The model under review builds one solid part; all positions refer to its coordinate system, in mm. A direction names the side the tool comes from. Coordinates: 2 decimals unless noted, no trailing zeros. Order: outer loops, then holes, each group sorted by start corner. A loop starts at its lowest first (then second) coordinate and runs counter-clockwise, first axis right, second up. Notation, with made-up numbers: M -25,23.5 L 4,23.5 A21 ccw 4,31.5 Z; hole C 50,26.5 d4. An arc over 180 degrees is marked long. Answer in a Markdown table with one row per item.
from build123d import *

# Parameters (mm, degrees)
SKETCH_1_W      = 27
SKETCH_1_H      = 27.6
SKETCH_1_W_2    = 23
SKETCH_1_H_2    = 1.5
EXTRUDE_1_DEPTH = 1.6
SKETCH_2_W      = 26.5
SKETCH_2_H      = 15
EXTRUDE_2_DEPTH = 1.5
SKETCH_3_W      = 5.6
SKETCH_3_H      = 12.6
EXTRUDE_3_DEPTH = 2
SKETCH_4_W      = 10.2
SKETCH_4_H      = 2.5
EXTRUDE_4_DEPTH = 2.5


with BuildPart() as part:
    # 草图1 → 凸台-拉伸1 (new body)
    with BuildSketch(Plane(origin=(0, 0, 0), x_dir=(1, 0, 0), z_dir=(0, 1, 0))):
        with Locations((13.5, -13.8)):
            Rectangle(SKETCH_1_W, SKETCH_1_H)
        with Locations((13.5, -26.05)):
            Rectangle(SKETCH_1_W_2, SKETCH_1_H_2, mode=Mode.SUBTRACT)
    extrude(amount=EXTRUDE_1_DEPTH)

    # 草图2 → 凸台-拉伸2 (add)
    with BuildSketch(Plane(origin=(0, 1.6, 0), x_dir=(1, 0, 0), z_dir=(0, 1, 0))):
        with Locations((13.5, -10.5)):
            Rectangle(SKETCH_2_W, SKETCH_2_H)
    extrude(amount=EXTRUDE_2_DEPTH)

    # 草图3 → 凸台-拉伸3 (add)
    with BuildSketch(Plane.XZ):
        with Locations((3.3, 6.9)):
            Rectangle(SKETCH_3_W, SKETCH_3_H)
    extrude(amount=EXTRUDE_3_DEPTH)

    # 草图4 → 凸台-拉伸4 (add)
    with BuildSketch(Plane.XZ):
        with Locations((13.5, 1.25)):
            Rectangle(SKETCH_4_W, SKETCH_4_H)
    extrude(amount=EXTRUDE_4_DEPTH)


solid = part.part
(1) Take a section at C-C (x = 3.75). Write out the cut boundary in (y, z).
Report:
| item | result |
|---|---|
| outline | M -2,0.6 L 0,0.6 L 0,0 L 1.6,0 L 1.6,3 L 3.1,3 L 3.1,18 L 1.6,18 L 1.6,25.3 L 0,25.3 L 0,13.2 L -2,13.2 Z; M 0,26.8 L 1.6,26.8 L 1.6,27.6 L 0,27.6 Z |
(2) To check wall thickness, follow line 1 (Z direction, x = 11.25, y = 0.05); line 2 (Z direction, x = 2, y = -0.6); line 3 (Y direction, x = 22, z = 24.75). State the ranges of each line that lie inside material, in increasing order. Write a range as [from, to].
Report:
| item | result |
|---|---|
| line 1 | [0, 25.3], [26.8, 27.6] |
| line 2 | [0.6, 13.2] |
| line 3 | [0, 1.6] |
(3) Insertion check: P1, Ø1.6, axis at x = 3, y = -1, coming from the -Z side; P2, Ø1.2, axis at y = 2.5, z = 8, coming from the -X side; P3, Ø3, axis at x = 2, z = 5.5, coming from the -Y side. Each pin has a flat end and moves straight along its axis. Give the tip position at first contact, or say it passes through.
Report:
| item | result |
|---|---|
| P1 | z = 0.6 |
| P2 | x = 0.25 |
| P3 | y = -2 |
(4) Take a section at B-B (y = -0.4). Write out the cut boundary in (x, z).
Report:
| item | result |
|---|---|
| outline | M 0.5,0.6 L 6.1,0.6 L 6.1,13.2 L 0.5,13.2 Z; M 8.4,0 L 18.6,0 L 18.6,2.5 L 8.4,2.5 Z |
(5) Take a section at D-D (z = 8.5). Write out the cut boundary in (x, y), then the cut area to 4 significant figures.
Report:
| item | result |
|---|---|
| outline | M 0,0 L 0.5,0 L 0.5,-2 L 6.1,-2 L 6.1,0 L 27,0 L 27,1.6 L 26.75,1.6 L 26.75,3.1 L 0.25,3.1 L 0.25,1.6 L 0,1.6 Z |
| area | 94.15 mm^2 |
(6) The part is to be moulded in two halves that separate along Z. For faces 1 (the flat face through (25, 1, 26)), 2 (the flat face through (13, 1, 26.8)), 3 (the flat face through (13, -1, 2.5)), 4 (the flat face through (6.1, -1, 7)), say which applies: +Z half, -Z half, draft (parallel to the pull), parting line (faces both ways), or undercut.
Report:
| item | result |
|---|---|
| face 1 | undercut |
| face 2 | undercut |
| face 3 | +Z half |
| face 4 | draft |
(7) Take a section at A-A (x = 9). Write out the cut boundary in (y, z).
Report:
| item | result |
|---|---|
| outline | M -2.5,0 L 1.6,0 L 1.6,3 L 3.1,3 L 3.1,18 L 1.6,18 L 1.6,25.3 L 0,25.3 L 0,2.5 L -2.5,2.5 Z; M 0,26.8 L 1.6,26.8 L 1.6,27.6 L 0,27.6 Z |
(8) Machinability: for faces 5 (the flat face through (13, 2, 18)), 6 (the flat face through (8.4, -1, 1)), 7 (the flat face through (0.25, 2, 11)), 8 (the flat face through (3, -1, 0.6)), which of the approach directions +Z, -Z, +X, -X, +Y, -Y give a long, thin tool a straight path to every point of the face, cutting with its end or side? Answer none if there is none.
Report:
| item | result |
|---|---|
| face 5 | +Z, +X, -X, +Y |
| face 6 | +Z, -Z, -Y |
| face 7 | +Z, -Z, -X, +Y |
| face 8 | -Z, -X, -Y |
